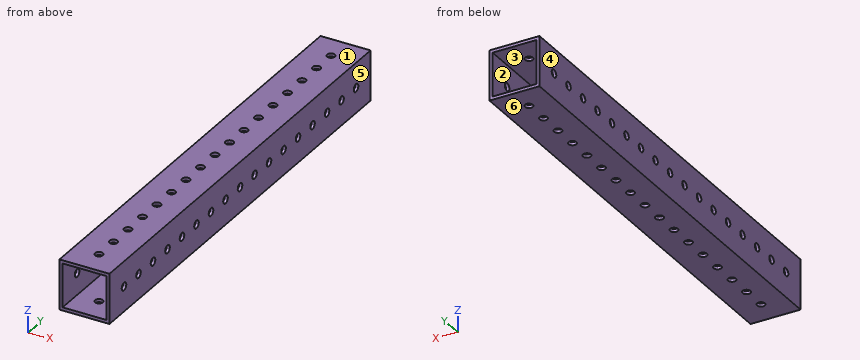
from build123d import *

# Parameters (mm, degrees)
SKETCH1_W                   = 25.4
SKETCH1_H                   = 25.4
SKETCH1_W_2                 = 22.225
SKETCH1_H_2                 = 22.225
BOSS_EXTRUDE1_DEPTH         = 228.6
F_22_0_157_DIAMETER_HOLE1_D = 3.9878
LPATTERN1_COUNT             = 17
LPATTERN1_PITCH             = 12.7
F_22_0_157_DIAMETER_HOLE2_D = 3.9878
LPATTERN2_COUNT             = 17
LPATTERN2_PITCH             = 12.7


with BuildPart() as part:
    # Sketch1 → Boss-Extrude1 (new body)
    with BuildSketch(Plane(origin=(0, 0, 0), x_dir=(1, 0, 0), z_dir=(0, 1, 0))):
        Rectangle(SKETCH1_W, SKETCH1_H)
        Rectangle(SKETCH1_W_2, SKETCH1_H_2, mode=Mode.SUBTRACT)
    extrude(amount=BOSS_EXTRUDE1_DEPTH)

    # #22 (0.157) Diameter Hole1 (through all)
    with Locations(Plane.XY.offset(12.7)):
        with Locations((0, 12.7)):
            f_22_0_157_diameter_hole1 = Hole(F_22_0_157_DIAMETER_HOLE1_D / 2)

    # LPattern1: #22 (0.157) Diameter Hole1 ×17
    with Locations(*[(0, i * LPATTERN1_PITCH, 0) for i in range(1, LPATTERN1_COUNT)]):
        add(f_22_0_157_diameter_hole1, mode=Mode.SUBTRACT)

    # #22 (0.157) Diameter Hole2 (through all)
    with Locations(Plane(origin=(12.7, 0, 0), x_dir=(0, 0, -1), z_dir=(1, 0, 0))):
        with Locations((0, 12.7)):
            f_22_0_157_diameter_hole2 = Hole(F_22_0_157_DIAMETER_HOLE2_D / 2)

    # LPattern2: #22 (0.157) Diameter Hole2 ×17
    with Locations(*[(0, i * LPATTERN2_PITCH, 0) for i in range(1, LPATTERN2_COUNT)]):
        add(f_22_0_157_diameter_hole2, mode=Mode.SUBTRACT)


solid = part.part
CAD build for the part. Positions are in the model's coordinates, mm. Face numbers are marked on the shaded views. A direction names the side the tool comes from. Round coordinates to 2 decimals unless told otherwise and drop trailing zeros. Loops run counter-clockwise (first coordinate to the right, second up) from the corner with the lowest first, then second, coordinate; pieces in that order, holes last.
(1) Drop a flat-ended pin along its axis: pin 1 (3 mm diameter, centred on y = 12.7, z = 0, fed in from +X). Give the stop position or say it passes through.
(2) Which spindle directions (+Z, -Z, +X, -X, +Y, -Y) get a long thin tool onto all of the face, cutting with end or side? Do the marked faces 1 and 2. Say none if no direction does.
(3) Cut at B-B (x = -4.5). Give the cut face in (y, z).
(4) Cut at A-A (y = 127). Give the cut face in (x, z), plus the area to 3 significant figures.
(5) Cut at C-C (z = 7.5). Give the cut face in (x, y).
(6) Wall check: line 1 along X through (y, z) = (79.5, -3); line 2 along Z through (x, y) = (-11.55, 190.5). Give the ranges that are in metal, low to high.
(7) Two-plate mould, pull along X, no slides. Class the marked faces 3, 4, 5 and 6: +X half, -X half, draft (parallel to the pull), parting line (faces both ways), or undercut.
Findings below:
1. pin 1: passes through
2. face 1: +Z, +X, -X, +Y, -Y
2. face 2: +Y, -Y
3. outline: (0, -12.7) - (228.6, -12.7) - (228.6, -11.11) - (0, -11.11) - close; (0, 11.11) - (228.6, 11.11) - (228.6, 12.7) - (0, 12.7) - close
4. outline: (-12.7, -12.7) - (-1.99, -12.7) - (-1.99, -11.11) - (-11.11, -11.11) - (-11.11, -1.99) - (-12.7, -1.99) - close; (-12.7, 1.99) - (-11.11, 1.99) - (-11.11, 11.11) - (-1.99, 11.11) - (-1.99, 12.7) - (-12.7, 12.7) - close; (1.99, -12.7) - (12.7, -12.7) - (12.7, -1.99) - (11.11, -1.99) - (11.11, -11.11) - (1.99, -11.11) - close; (1.99, 11.11) - (11.11, 11.11) - (11.11, 1.99) - (12.7, 1.99) - (12.7, 12.7) - (1.99, 12.7) - close
4. area: 126 mm2
5. outline: (-12.7, 0) - (-11.11, 0) - (-11.11, 228.6) - (-12.7, 228.6) - close; (11.11, 0) - (12.7, 0) - (12.7, 228.6) - (11.11, 228.6) - close
6. line 1: x = -12.7 to -11.11, 11.11 to 12.7
6. line 2: z = -12.7 to -1.99, 1.99 to 12.7
7. face 3: undercut
7. face 4: -X half
7. face 5: +X half
7. face 6: draft
